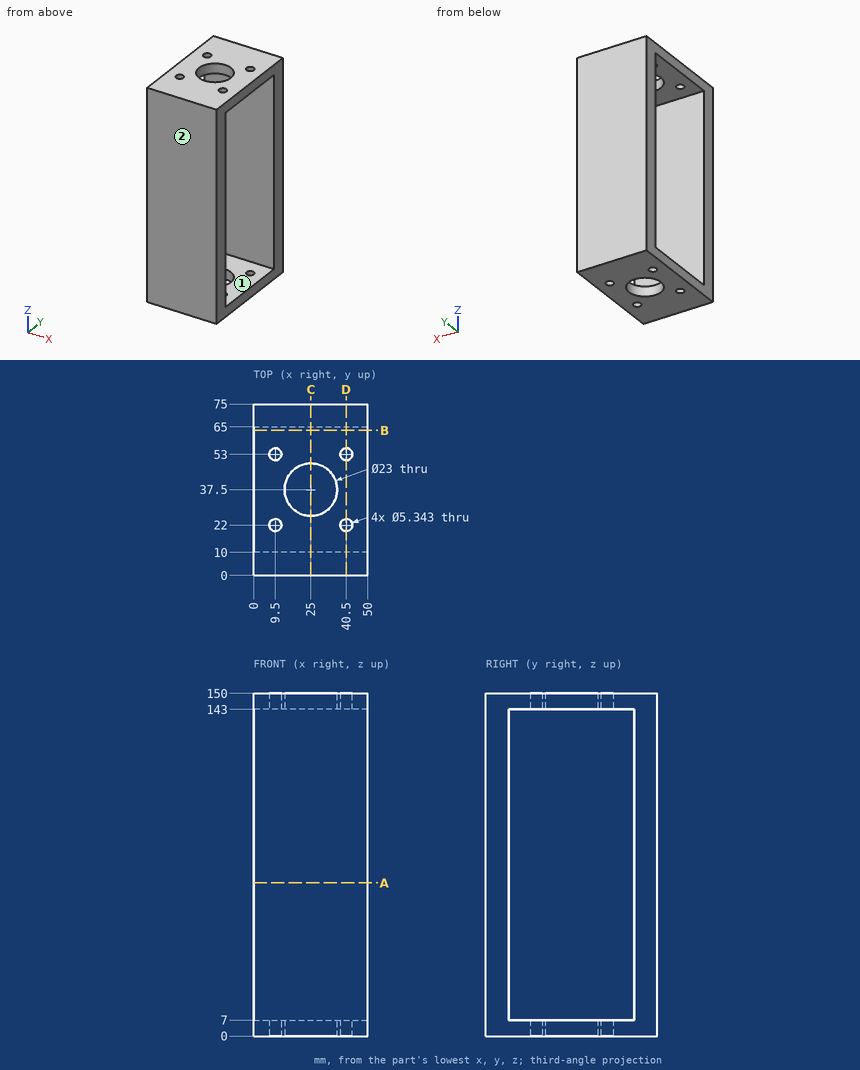
Geometry: see drawing. Coordinates: mm, zero at the bounding-box minimum. A direction names the side the tool comes from. Give positions to 0.01 mm unless a question says otherwise; leave off trailing zeros. Loops run counter-clockwise (first coordinate to the right, second up) from the corner with the lowest first, then second, coordinate; pieces in that order, holes last. Notation, with made-up numbers: (58, -7.75) - (67, -7.75) arc R28 ccw to (67, 14.25) - close; hole circle Ø4 at (54, 42). An arc over 180 degrees is marked (long way). Use CSV: the item, a comma, the result in double quotes. Start each with the question number.
1. Pin query (flat end, axial travel): pin 1 (8.5 mm diameter, centred on x = 9.5, y = 53, fed in from -Z). Return the tip coordinate at first contact, or that it passes through.
2. Reachability of the marked faces 1 and 2 from +Z, -Z, +X, -X, +Y, -Y: full face, straight path, thin tool, end or side. Return the list, or none.
3. Section C-C (x = 25). Output: boundary loops of the cut face in (y, z).
4. Section B-B (y = 63.5). Output: boundary loops of the cut face in (x, z).
5. Section D-D (x = 40.5). Output: boundary loops of the cut face in (y, z), then the cut area to 3 significant figures.
6. Ray query, L1, parallel to X at y = 53, z = 148; L2, parallel to Y at x = 40.5, z = 148; L3, parallel to Y at x = 22, z = 123.5. Return the intervals inside material, ascending.
7. Section A-A (z = 67). Output: boundary loops of the cut face in (x, y), then the cut area to 3 significant figures.
Response:
1,pin 1,"z = 0"
2,face 1,"+X, -X"
2,face 2,"+Z, -Z, +X, -X, -Y"
3,outline,"(0, 0) - (26, 0) - (26, 7) - (10, 7) - (10, 143) - (26, 143) - (26, 150) - (0, 150) - close; (49, 0) - (75, 0) - (75, 150) - (49, 150) - (49, 143) - (65, 143) - (65, 7) - (49, 7) - close"
4,outline,"(0, 0) - (50, 0) - (50, 7) - (0, 7) - close; (0, 143) - (50, 143) - (50, 150) - (0, 150) - close"
5,outline,"(0, 0) - (19.33, 0) - (19.33, 7) - (10, 7) - (10, 143) - (19.33, 143) - (19.33, 150) - (0, 150) - close; (24.67, 0) - (50.33, 0) - (50.33, 7) - (24.67, 7) - close; (24.67, 143) - (50.33, 143) - (50.33, 150) - (24.67, 150) - close; (55.67, 0) - (75, 0) - (75, 150) - (55.67, 150) - (55.67, 143) - (65, 143) - (65, 7) - (55.67, 7) - close"
5,area,"3,620 mm²"
6,L1,"0 to 6.83, 12.17 to 37.83, 43.17 to 50"
6,L2,"0 to 19.33, 24.67 to 50.33, 55.67 to 75"
6,L3,"0 to 10, 65 to 75"
7,outline,"(0, 0) - (50, 0) - (50, 10) - (0, 10) - close; (0, 65) - (50, 65) - (50, 75) - (0, 75) - close"
7,area,"1,000 mm²"
